```python
from build123d import *

# Parameters (mm, degrees)
SKETCH1_R           = 1.651
SKETCH1_R_2         = 11.07313
BOSS_EXTRUDE1_DEPTH = 2
BOSS_EXTRUDE2_DEPTH = 2
FILLET2_R           = 2
FILLET3_R           = 2


with BuildPart() as part:
    # Sketch1 → Boss-Extrude1 (new body)
    with BuildSketch(Plane.XY):
        with BuildLine():
            Line((-17.78, -10.602028155), (-17.78, 20.701))
            Line((-17.78, 20.701), (17.78, 20.701))
            Line((17.78, 20.701), (17.78, -10.602028155))
            ThreePointArc((17.78, -10.602028155), (0, -20.701), (-17.78, -10.602028155))
        make_face()
        with Locations((-12.515790027, -12.515790027)):
            Circle(SKETCH1_R, mode=Mode.SUBTRACT)
        with Locations((12.515790027, -12.515790027)):
            Circle(SKETCH1_R, mode=Mode.SUBTRACT)
        with Locations((12.515790027, 12.515790027)):
            Circle(SKETCH1_R, mode=Mode.SUBTRACT)
        with Locations((-12.515790027, 12.515790027)):
            Circle(SKETCH1_R, mode=Mode.SUBTRACT)
        Circle(SKETCH1_R_2, mode=Mode.SUBTRACT)
    boss_extrude1 = extrude(amount=BOSS_EXTRUDE1_DEPTH)

    # Mirror1: Boss-Extrude1 across plane
    add(boss_extrude1.mirror(Plane(origin=(0, 9.3505, -9.3505), x_dir=(0, 0.7071067811865465, 0.7071067811865486), z_dir=(0, -0.7071067811865488, 0.7071067811865464))))

    # Sketch2 → Boss-Extrude2 (add)
    with BuildSketch(Plane.ZY.offset(17.78)):
        Polygon((0, -10.602028155), (-29.303028155, 18.701), (0, 18.701), align=None)
    boss_extrude2 = extrude(amount=-BOSS_EXTRUDE2_DEPTH)

    # Mirror2: Boss-Extrude2 across plane
    add(boss_extrude2.mirror(Plane(origin=(0, 0, 0), x_dir=(0, 0, 1), z_dir=(1, 0, 0))))

    # Fillet2
    fillet2_edges = [part.edges().sort_by_distance(p)[0] for p in [
        (-11.07313, 0, 0),
        (-11.07313, 18.701, -18.701),
    ]]
    fillet(fillet2_edges, radius=FILLET2_R - 0.0001)  # a hair under: the kernel refuses the full size

    # Fillet3
    fillet3_edges = [part.edges().sort_by_distance(p)[0] for p in [
        (-16.78, -10.602028155, 0),
        (-16.78, 18.701, -29.303028155),
        (16.78, -10.602028155, 0),
        (16.78, 18.701, -29.303028155),
    ]]
    fillet(fillet3_edges, radius=FILLET3_R)


solid = part.part
```
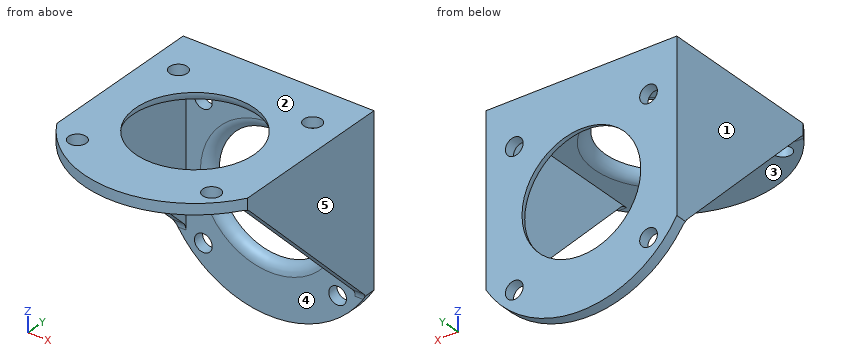
Input: part model. Units: mm. Frame: model coordinates. Face numbers are marked on the shaded views. A direction names the side the tool comes from. Coordinates: 2 decimals unless noted, no trailing zeros.
Q1. Mould query, pull axis X, two halves, no side actions, for the marked faces 1, 2 and 3. Classes: +X half, -X half, draft (parallel to the pull), parting line (faces both ways), or undercut.
Results are:
face 1: -X half
face 2: draft
face 3: undercut
Q2. Contact query for flat-ended pins moving along their axis: pin 1 (5.5 mm diameter, centred on x = -12.52, z = -6.19, fed in from +Y); pin 2 (17.5 mm diameter, centred on x = 7, z = -18.5, fed in from -Y); pin 3 (3 mm diameter, centred on x = 12.52, y = -12.52, fed in from +Z); pin 4 (5.5 mm diameter, centred on x = -12.52, y = -12.52, fed in from -Z). Output: stop coordinate, or through.
Results are:
pin 1: stops at y = 20.7
pin 2: stops at y = 18.7
pin 3: passes through
pin 4: stops at z = 0
Q3. Line query: line 1 along X through (y, z) = (9.5, -17.5); line 2 along Y through (x, z) = (-15, -15); line 3 along Z through (x, y) = (14, -2.5). Output: solid intervals per line, ascending.
Results are:
line 1: x = -17.78 to -15.78, 15.78 to 17.78
line 2: y = 18.7 to 20.7
line 3: z = 0 to 2
Q4. Section B-B, the plane x = 0. Give the number of separate pieces and of enclosed holes in the cut face, and give its area (3 significant figures).
Results are:
separate pieces: 3
enclosed holes: 0
area: 69.6 mm2
Q5. Set-up query: the marked faces 4 and 5. Return all of +Z, -Z, +X, -X, +Y, -Y with unobstructed straight access to the full face (end or side cutting, diameter ignored); none if empty.
Results are:
face 4: -Z, -Y
face 5: +Z, -Z, +X, +Y, -Y
